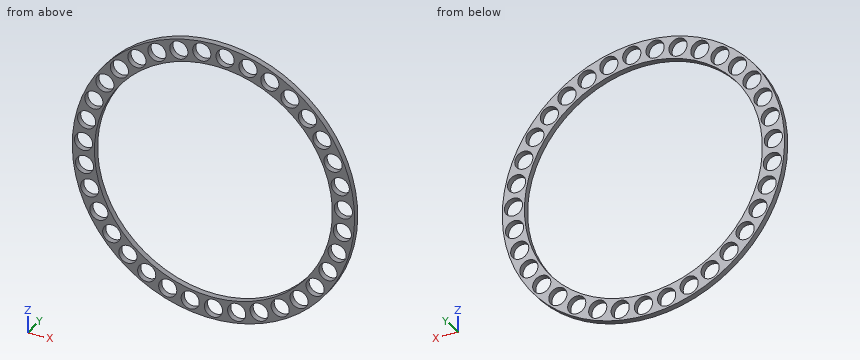
```python
from build123d import *

# Parameters (mm, degrees)
CROQUIS1_R              = 70
CROQUIS1_R_2            = 59
SALIENTE_EXTRUIR1_DEPTH = 1.5
CROQUIS3_R              = 4.5
CORTAR_EXTRUIR1_DEPTH   = 5
MATRIZC1_COUNT          = 35


with BuildPart() as part:
    # Croquis1 → Saliente-Extruir1 (new, symmetric)
    with BuildSketch(Plane(origin=(0, 0, 0), x_dir=(1, 0, 0), z_dir=(0, 1, 0))):
        with Locations(Location((0, 0, 0), (0, 0, 270))):
            Circle(CROQUIS1_R)
        with Locations(Location((0, 0, 0), (0, 0, 270))):
            Circle(CROQUIS1_R_2, mode=Mode.SUBTRACT)
    extrude(amount=SALIENTE_EXTRUIR1_DEPTH, both=True)

    # Croquis3 → Cortar-Extruir1 (cut)
    with BuildSketch(Plane(origin=(0, -1.5, 0), x_dir=(-1, 0, 0), z_dir=(0, -1, 0))):
        with Locations(Location((0, 64.5, 0), (0, 0, 90))):
            Circle(CROQUIS3_R)
    cortar_extruir1 = extrude(amount=-CORTAR_EXTRUIR1_DEPTH, mode=Mode.SUBTRACT)

    # MatrizC1: Cortar-Extruir1 ×35 about axis
    matrizc1_axis = Axis((0, 0, 0), (0, 1, 0))
    for i in range(1, MATRIZC1_COUNT):
        add(cortar_extruir1.rotate(matrizc1_axis, i * 360 / MATRIZC1_COUNT), mode=Mode.SUBTRACT)


solid = part.part
```
Work out the finished part from the listing and answer in its coordinate system (mm). Give positions to 0.01 mm unless a question says otherwise; leave off trailing zeros. Order: outer loops, then holes, each group sorted by start corner. A loop starts at its lowest first (then second) coordinate and runs counter-clockwise, first axis right, second up. Notation, with made-up numbers: M 62.5,28 L 118.5,28 A20 ccw 118.5,33 Z; hole C -35.5,-30 d3. An arc over 180 degrees is marked long. Return JSON: item names as keys, results as strings.
1) Section B-B, the plane y = 0.65 is taken. Give the number of separate pieces and of enclosed holes in the cut face, plus the area to 3 significant figures.
Resolved:
{"separate pieces": "1", "enclosed holes": "36", "area": "2,230 mm^2"}
2) Section A-A, the plane z = 0 is taken. Write down the section's boundary in (x, y), plus the area to 3 significant figures.
Resolved:
{"outline": "M -70,-1.5 L -67.88,-1.5 L -67.88,1.5 L -70,1.5 Z; M -60.99,-1.5 L -59,-1.5 L -59,1.5 L -60.99,1.5 Z; M 59,-1.5 L 60.99,-1.5 L 60.99,1.5 L 59,1.5 Z; M 67.88,-1.5 L 70,-1.5 L 70,1.5 L 67.88,1.5 Z", "area": "24.6 mm^2"}
3) Each of these flat-tipped pins is pushed along its axis until it touches: pin 1 (11.5 mm diameter, centred on x = 56.8, z = -30.56, fed in from +Y); pin 2 (8 mm diameter, centred on x = -53.83, z = 35.53, fed in from -Y); pin 3 (1.5 mm diameter, centred on y = -1, z = -37, fed in from -X). Where does it stop, or does it pass through?
Resolved:
{"pin 1": "y = 1.5", "pin 2": "through", "pin 3": "x = -59.88"}
4) Straight lines are drawn through the part: line 1 along X through (y, z) = (-0.8, -12); line 2 along X through (y, z) = (-0.85, 13.5); line 3 along Z through (x, y) = (-2.5, -0.25). For each, find the intervals that lie inside material, in ascending order. Write a range as [from, to].
Resolved:
{"line 1": "[-68.96, -66.93], [-60.9, -57.77], [57.77, 60.9], [66.93, 68.96]", "line 2": "[-68.69, -67.3], [-58.46, -57.43], [57.43, 58.46], [67.3, 68.69]", "line 3": "[-69.96, -68.24], [-60.76, -58.95], [58.95, 61.16], [67.32, 69.96]"}
